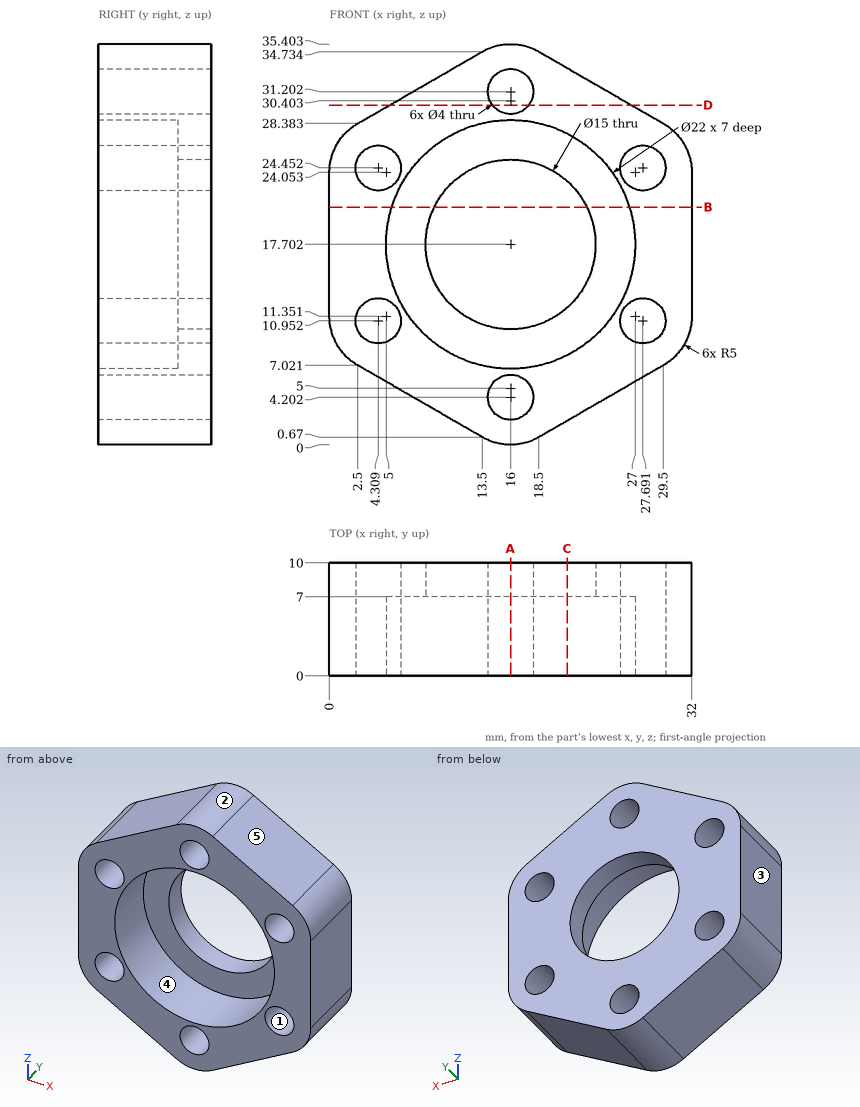
Answer from the drawing. Dimensions are ordinates in mm from the lowest x, y and z of the part. A direction names the side the tool comes from. Coordinates: 2 decimals unless noted, no trailing zeros. Order: outer loops, then holes, each group sorted by start corner. A loop starts at its lowest first (then second) coordinate and runs counter-clockwise, first axis right, second up. Notation, with made-up numbers: (14.25, 22) - (46.25, 22) arc R35 cw to (46.25, 60) - close; hole circle Ø3 at (-18.5, 84). An arc over 180 degrees is marked (long way). Answer as a JSON object with one key per item and string values. Group by question number.
Item 1: A tool of negligible diameter and unlimited length cuts with its end or side. For the marked faces 4 and 5, from which of +Z, -Z, +X, -X, +Y, -Y can it reach the whole face along a straight path? Write none if from no direction.
Item 2: Section B-B (z = 21) is taken. Give the vertices of the cut face in (x, y) (1 decimal), plus the area to 3 significant figures.
Item 3: Section C-C (x = 21) is taken. Give the vertices of the cut face in (y, z).
Item 4: Section D-D (z = 30) is taken. Give the vertices of the cut face in (x, y), plus the area to 3 significant figures.
Item 5: Consider probe 1 along Z at (x, y) = (29.5, 8.25) (1 decimal); probe 2 along X at (y, z) = (9.75, 18) (1 decimal); probe 3 along X at (y, z) = (1.75, 24) (1 decimal). Determine where each line is inside the solid, lowest interval first. Write a range as from..to.
Item 6: Section A-A (x = 16) is taken. Give the vertices of the cut face in (y, z).
Item 7: The mould has two halves that part along X. Classify the marked faces 1, 2 and 3: +X half, -X half, draft (parallel to the pull), parting line (faces both ways), or undercut.
Item 8: Flat-ended cylindrical pins translate along their axes: P1, Ø4.5, axis at x = 27.69, z = 24.45, coming from the +Y side; P2, Ø3.5, axis at x = 4.31, z = 10.95, coming from the +Y side; P3, Ø11, axis at x = 19, z = 22, coming from the -Y side; P4, Ø6, axis at x = 25.5, y = 4.5, coming from the +Z side (1 decimal). Find the tip coordinate at first contact, or state that the pin passes through.
Results are:
{
 "1": {"face 4": "-Y", "face 5": "+Z, +X, +Y, -Y"},
 "2": {"outline": "(0, 0) - (5.5, 0) - (5.5, 7) - (9.3, 7) - (9.3, 10) - (0, 10) - close; (22.7, 7) - (26.5, 7) - (26.5, 0) - (32, 0) - (32, 10) - (22.7, 10) - close", "area": "133 mm^2"},
 "3": {"outline": "(0, 2.11) - (10, 2.11) - (10, 12.11) - (7, 12.11) - (7, 7.9) - (0, 7.9) - close; (0, 27.5) - (7, 27.5) - (7, 23.29) - (10, 23.29) - (10, 33.29) - (0, 33.29) - close"},
 "4": {"outline": "(5.3, 0) - (14.4, 0) - (14.4, 10) - (5.3, 10) - close; (17.6, 0) - (26.7, 0) - (26.7, 10) - (17.6, 10) - close", "area": "182 mm^2"},
 "5": {"probe 1": "z = 7..10.1, 11.8..23.6, 25.3..28.4", "probe 2": "x = 0..8.5, 23.5..32", "probe 3": "x = 0..2.4, 6.3..7, 25..25.7, 29.6..32"},
 "6": {"outline": "(0, 0) - (10, 0) - (10, 2.2) - (0, 2.2) - close; (0, 6.2) - (10, 6.2) - (10, 10.2) - (7, 10.2) - (7, 6.7) - (0, 6.7) - close; (0, 28.7) - (7, 28.7) - (7, 25.2) - (10, 25.2) - (10, 29.2) - (0, 29.2) - close; (0, 33.2) - (10, 33.2) - (10, 35.4) - (0, 35.4) - close"},
 "7": {"face 1": "undercut", "face 2": "parting line", "face 3": "-X half"},
 "8": {"P1": "stops at y = 10", "P2": "passes through", "P3": "stops at y = 7", "P4": "stops at z = 32.4"}
}
